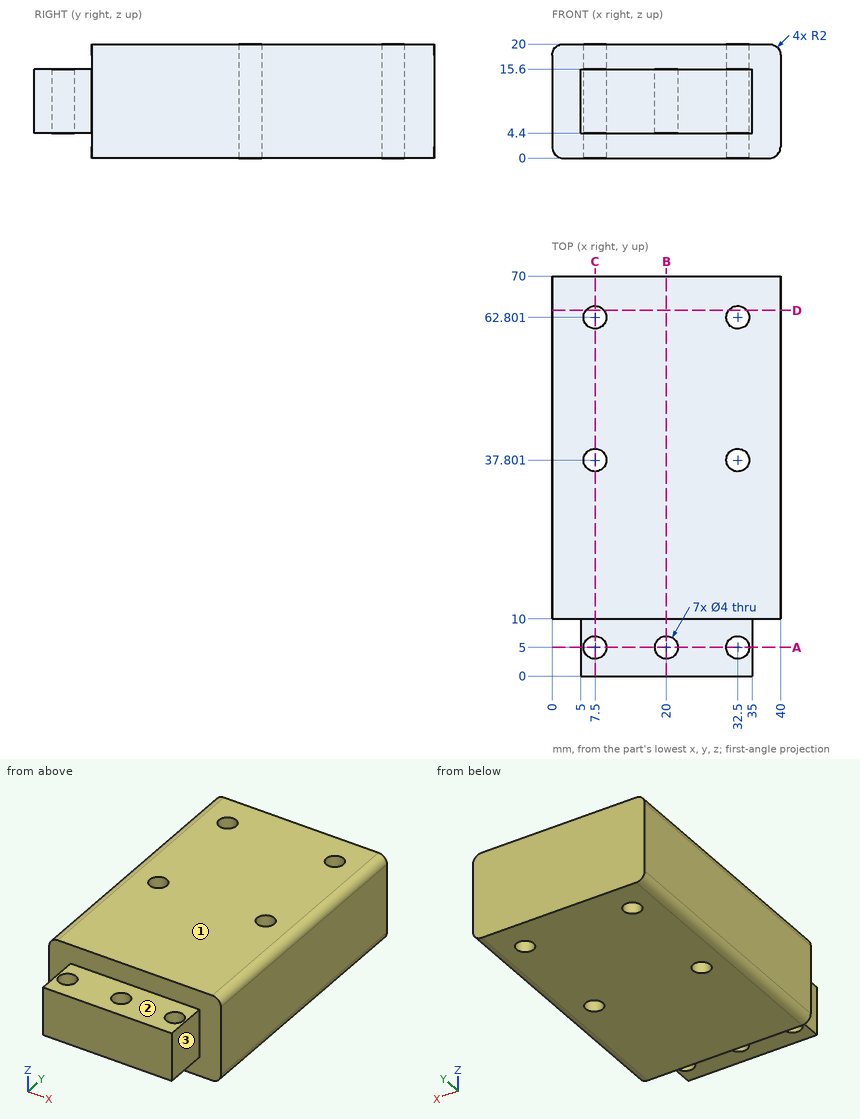
For this review, use the dimensioned drawing (mm, ordinates from the lowest corner) and the shaded views. A direction names the side the tool comes from. Give positions to 0.01 mm unless a question says otherwise; leave off trailing zeros. Order: outer loops, then holes, each group sorted by start corner. A loop starts at its lowest first (then second) coordinate and runs counter-clockwise, first axis right, second up. Notation, with made-up numbers: (-22, -15) - (-1, -15) arc R9 cw to (-1, 0) - close; hole circle Ø4 at (56, -33.75). An arc over 180 degrees is marked (long way). Use CSV: the item, a comma, the result in double quotes. Start each with the question number.
Q1. We need section C-C, the plane x = 7.5. Write out the cut boundary in (y, z), and give its area (3 significant figures).
Q2. To check wall thickness, follow line 1 along Y through (x, z) = (7.5, 9); line 2 along Y through (x, z) = (32, 5.25); line 3 along X through (y, z) = (4, 13.5). State the ranges of each line that lie inside material, in increasing order. Write a range as [from, to].
Q3. We need section B-B, the plane x = 20. Write out the cut boundary in (y, z).
Q4. We need section A-A, the plane y = 5. Write out the cut boundary in (x, z).
Q5. Tool access review of the marked faces 1, 2 and 3: name each direction out of +Z, -Z, +X, -X, +Y, -Y from which nothing blocks a thin tool from reaching the whole face with its end or side.
Q6. We need section D-D, the plane y = 64. Write out the cut boundary in (x, z).
Q7. Clearance check with flat-ended pins moving along their axes: pin 1 Ø3 at (x, y) = (20, 5) entering from -Z; pin 2 Ø5 at (x, y) = (26.5, 6) entering from +Z; pin 3 Ø6.5 at (x, y) = (32.5, 5) entering from -Z. State where each tip first meets the part, or that it passes through.
Outcome:
1,outline,"(0, 4.4) - (3, 4.4) - (3, 15.6) - (0, 15.6) - close; (7, 4.4) - (10, 4.4) - (10, 0) - (35.8, 0) - (35.8, 20) - (10, 20) - (10, 15.6) - (7, 15.6) - close; (39.8, 0) - (60.8, 0) - (60.8, 20) - (39.8, 20) - close; (64.8, 0) - (70, 0) - (70, 20) - (64.8, 20) - close"
1,area,"1,110 mm^2"
2,line 1,"y = [0, 3], [7, 35.8], [39.8, 60.8], [64.8, 70]"
2,line 2,"y = [0, 3.06], [6.94, 35.86], [39.74, 60.86], [64.74, 70]"
2,line 3,"x = [5, 5.77], [9.23, 18.27], [21.73, 30.77], [34.23, 35]"
3,outline,"(0, 4.4) - (3, 4.4) - (3, 15.6) - (0, 15.6) - close; (7, 4.4) - (10, 4.4) - (10, 0) - (70, 0) - (70, 20) - (10, 20) - (10, 15.6) - (7, 15.6) - close"
4,outline,"(5, 4.4) - (5.5, 4.4) - (5.5, 15.6) - (5, 15.6) - close; (9.5, 4.4) - (18, 4.4) - (18, 15.6) - (9.5, 15.6) - close; (22, 4.4) - (30.5, 4.4) - (30.5, 15.6) - (22, 15.6) - close; (34.5, 4.4) - (35, 4.4) - (35, 15.6) - (34.5, 15.6) - close"
5,face 1,"+Z, +X, -X, +Y, -Y"
5,face 2,"+Z, +X, -X, -Y"
5,face 3,"+Z, -Z, +X, -Y"
6,outline,"(0, 2) arc R2 ccw to (2, 0) - (5.9, 0) - (5.9, 20) - (2, 20) arc R2 ccw to (0, 18) - close; (9.1, 0) - (30.9, 0) - (30.9, 20) - (9.1, 20) - close; (34.1, 0) - (38, 0) arc R2 ccw to (40, 2) - (40, 18) arc R2 ccw to (38, 20) - (34.1, 20) - close"
7,pin 1,"passes through"
7,pin 2,"stops at z = 15.6"
7,pin 3,"stops at z = 4.4"
